Design review of the part built by this model. Coordinates are the model's own, in mm. Face numbers are marked on the shaded views. A direction names the side the tool comes from. Coordinates: 2 decimals unless noted, no trailing zeros. Write each loop counter-clockwise with the first axis right and the second up, starting at its lowest first coordinate (ties: lowest second). Pieces come first, ordered by that corner, then holes.
Q1. Insertion check: pin 1 (1 mm diameter, centred on x = 5, y = 22, fed in from -Z); pin 2 (6 mm diameter, centred on x = 2, z = -6, fed in from +Y); pin 3 (5 mm diameter, centred on x = 3.5, z = 8.5, fed in from -Y). Each pin has a flat end and moves straight along its axis. Give the tip position at first contact, or say it passes through.
Q2. Machinability: for the marked faces 4, 5 and 6, which of the approach directions +Z, -Z, +X, -X, +Y, -Y give a long, thin tool a straight path to every point of the face, cutting with its end or side? Answer none if there is none.
Q3. Mouldability with a two-part tool opening along X and no side actions: class the marked faces 1, 2 and 3 as pulls with the +X half, pulls with the -X half, needs draft (parallel to the pull), parting line crosses it, or undercut.
Q4. Take a section at C-C (x = 8.5). Give the boundary of the cut face in (y, z).
Q5. For probe 1 along Z at (x, y) = (8, 19.5); probe 2 along X at (y, z) = (14, -11), list the stretches that pass through material, from the lowest coordinate up.
Q6. Take a section at B-B (y = 18.5). Give the boundary of the cut face in (x, z).
Q7. Take a section at A-A (z = -1). Give the boundary of the cut face in (x, y), and give its area (3 significant figures).
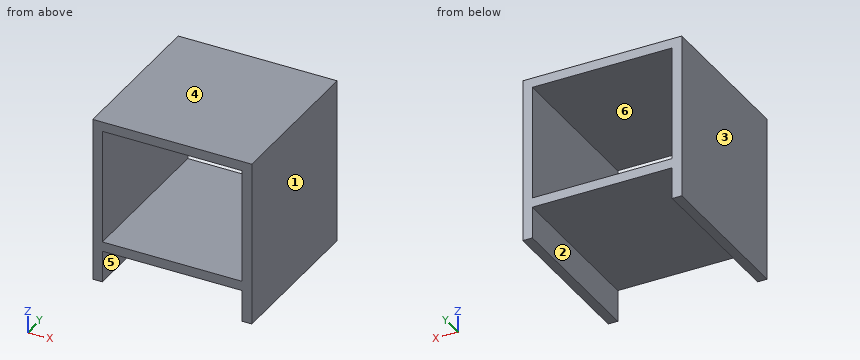
```python
from build123d import *

# Parameters (mm, degrees)
EXTRUDE_1_DEPTH = 25


with BuildPart() as part:
    # Эскиз1 → Бобышка-Вытянуть1 (new body)
    with BuildSketch(Plane(origin=(0, 0, 0), x_dir=(1, 0, 0), z_dir=(0, 1, 0))):
        Polygon((11, 8), (-11, 8), (-11, 13), (-12.5, 13), (-12.5, 6), (-12.5, -11), (-12.5, -11.5), (-12.5, -13), (-11, -13), (11, -13), (12.5, -13), (12.5, -11.5), (12.5, 6), (12.5, 6.5), (12.5, 8), (12.5, 13), (11, 13), align=None)
        Polygon((-11, 6.5), (11, 6.5), (11, 6), (11, -11), (11, -11.5), (-11, -11.5), (-11, -11), (-11, 6), align=None, mode=Mode.SUBTRACT)
    extrude(amount=EXTRUDE_1_DEPTH)


solid = part.part
```
Response:
1. pin 1: stops at z = -8
1. pin 2: stops at y = 25
1. pin 3: passes through
2. face 4: +Z, +X, -X, +Y, -Y
2. face 5: -Z, +Y, -Y
2. face 6: +Y, -Y
3. face 1: pulls with the +X half
3. face 2: undercut
3. face 3: pulls with the -X half
4. outline: (0, -8) - (25, -8) - (25, -6.5) - (0, -6.5) - close; (0, 11.5) - (25, 11.5) - (25, 13) - (0, 13) - close
5. probe 1: z = -8 to -6.5, 11.5 to 13
5. probe 2: x = -12.5 to -11, 11 to 12.5
6. outline: (-12.5, -13) - (-11, -13) - (-11, -8) - (11, -8) - (11, -13) - (12.5, -13) - (12.5, 13) - (-12.5, 13) - close; hole (-11, -6.5) - (11, -6.5) - (11, 11.5) - (-11, 11.5) - close
7. outline: (-12.5, 0) - (-11, 0) - (-11, 25) - (-12.5, 25) - close; (11, 0) - (12.5, 0) - (12.5, 25) - (11, 25) - close
7. area: 75.0 mm2
